from build123d import *
from build123d.topology import SkipClean

# Parameters (mm, degrees)
SKETCH_1_R               = 8
EXTRUDE_1_DEPTH          = 17
SKETCH_2_R               = 30
EXTRUDE_2_DEPTH          = 3
CUT_EXTRUDE_1_DEPTH      = 47.904158
CUT_EXTRUDE_2_DEPTH      = 50.558047
CUT_EXTRUDE_2_DEPTH_BACK = 50.558047
SKETCH_4_R               = 1.15
EXTRUDE_START            = 15
EXTRUDE_3_DEPTH          = 15
FILLET_1_R               = 3
CUT_EXTRUDE_3_DEPTH      = 46.70558
CUT_EXTRUDE_3_DEPTH_BACK = 46.70558
SKETCH_6_R               = 1.25


with BuildPart() as part:
    # 草图1 → 凸台-拉伸1 (new body)
    with BuildSketch(Plane(origin=(0, 0, 0), x_dir=(1, 0, 0), z_dir=(0, 1, 0))):
        with Locations(Location((0, 0, 0), (0, 0, 270))):
            Circle(SKETCH_1_R)
    extrude(amount=EXTRUDE_1_DEPTH)

    # 草图2 → 凸台-拉伸2 (add)
    with BuildSketch(Plane(origin=(0, 17, 0), x_dir=(1, 0, 0), z_dir=(0, 1, 0))):
        with Locations(Location((0, 0, 0), (0, 0, 270))):
            Circle(SKETCH_2_R)
    extrude(amount=EXTRUDE_2_DEPTH)

    # 草图3 → 切除-拉伸1 (cut, through all)
    with BuildSketch(Plane.XZ):
        with BuildLine():
            Line((-4, 3), (-4, -3))
            ThreePointArc((-4, -3), (5, 0), (-4, 3))
        make_face()
    extrude(amount=-CUT_EXTRUDE_1_DEPTH, mode=Mode.SUBTRACT)

    # 草图4 → 切除-拉伸2 (cut, two sides: drawn at the far end of the back side and taken through both)
    with BuildSketch(Plane(origin=(-4, 0, 0), x_dir=(0, 0, -1), z_dir=(1, 0, 0)).offset(-CUT_EXTRUDE_2_DEPTH_BACK)):
        with Locations((0, 10)):
            Circle(SKETCH_4_R)
    extrude(amount=CUT_EXTRUDE_2_DEPTH + CUT_EXTRUDE_2_DEPTH_BACK, mode=Mode.SUBTRACT)

    # 草图5 → 凸台-拉伸3 (add)
    with SkipClean():  # the faces are left unmerged after this step: merging them gives an invalid solid
        with BuildSketch(Plane.XZ.offset(-17).offset(EXTRUDE_START)):
            with BuildLine():
                Line((-2, 29.933259), (-2, 20))
                Line((-2, 20), (2, 20))
                Line((2, 20), (2, 29.933259))
                ThreePointArc((2, 29.933259), (0, 30), (-2, 29.933259))
            make_face()
        extrude(amount=-EXTRUDE_3_DEPTH)

    # 圆角1
    fillet_1_edges = [part.edges().sort_by_distance(p)[0] for p in [
        (0, 17, -8),
    ]]
    fillet(fillet_1_edges, radius=FILLET_1_R)

    # 草图6 → 切除-拉伸3 (cut, two sides: drawn at the far end of the back side and taken through both)
    with SkipClean():  # the faces are left unmerged after this step: merging them gives an invalid solid
        with BuildSketch(Plane.XZ.offset(-17).offset(-CUT_EXTRUDE_3_DEPTH_BACK)):
            with Locations(Location((-16, 0, 0), (0, 0, 270))):
                Circle(SKETCH_6_R)
            with Locations(Location((16, 0, 0), (0, 0, 90))):
                Circle(SKETCH_6_R)
        extrude(amount=CUT_EXTRUDE_3_DEPTH + CUT_EXTRUDE_3_DEPTH_BACK, mode=Mode.SUBTRACT)


solid = part.part
Verification items for the finished model (mm, model axes). A direction names the side the tool comes from. Coordinates: 2 decimals unless noted, no trailing zeros. Write each loop counter-clockwise with the first axis right and the second up, starting at its lowest first coordinate (ties: lowest second). Pieces come first, ordered by that corner, then holes. Notation, with made-up numbers: M 70,-20.5 L 114,-20.5 A10 cw 114,-14.5 Z; hole C -39.5,46 d4. An arc over 180 degrees is marked long. Use CSV: the item, a comma, the result in double quotes.
Q1. Go/stop test with flat-tipped pins: P1, Ø1, axis at x = 7.5, y = 9, coming from the -Z side; P2, Ø4, axis at x = -16, z = 0, coming from the -Y side; P3, Ø10, axis at y = 17, z = 10, coming from the +X side. Record where each tip stops, or that it passes through.
Computed values:
P1,"z = -3.87"
P2,"y = 17"
P3,"x = 29.58"
Q2. Section check A-A, the plane z = 0. State how many separate pieces and enclosed holes the cut face has, and give its area (3 significant figures).
Computed values:
separate pieces,"6"
enclosed holes,"0"
area,"245 mm²"
Q3. Set-up check for faces 4 (the flat face through (2, 9, 25)), 5 (the cylindrical face through (-7.81, 6.9, -1.73)), 6 (the flat face through (-2, 9, 25)), 7 (the flat face through (0, 2, 25)), 8 (the flat face through (-4, 9.9, -1.3)): record each of +Z, -Z, +X, -X, +Y, -Y from which the full face is reachable in a straight line by a thin tool's end or side.
Computed values:
face 4,"+Z, +X, -Y"
face 5,"-Y"
face 6,"+Z, -X, -Y"
face 7,"+Z, +X, -X, -Y"
face 8,"+Y, -Y"
Q4. Section check B-B, the plane x = 0. Enter the section's corners in (y, z).
Computed values:
outline,"M 0,-8 L 14,-8 A3 cw 17,-11 L 17,-30 L 20,-30 L 20,-5 L 0,-5 Z; M 0,5 L 20,5 L 20,30 L 2,30 L 2,20 L 17,20 L 17,11 A3 cw 14,8 L 0,8 Z"
Q5. Section check D-D, the plane y = 10. Enter the section's corners in (x, z), and give its area (3 significant figures).
Computed values:
outline,"M -7.92,-1.15 A8 ccw 7.92,-1.15 L 4.87,-1.15 A5 cw -4,-3 L -4,-1.15 Z; M -7.92,1.15 L -4,1.15 L -4,3 A5 cw 4.87,1.15 L 7.92,1.15 A8 ccw Z; M -2,20 L 2,20 L 2,29.93 A30 ccw -2,29.93 Z"
area,"150 mm²"
Q6. Mould release check, pull along Y, two halves, no side actions. Record for faces 1 (the cylindrical face through (6.41, 8.877, 0.249)), 2 (the flat face through (-5, 0, 0)), 3 (the flat face through (0, 9, 20)): pulls with the +Y half, pulls with the -Y half, needs draft (parallel to the pull), parting line crosses it, or undercut.
Computed values:
face 1,"undercut"
face 2,"pulls with the -Y half"
face 3,"needs draft"
Q7. Thickness scan on line 1 along X through (y, z) = (18.3, 0); line 2 along X through (y, z) = (17.75, -1); line 3 along Y through (x, z) = (9.5, 22). Record the ranges inside material, lowest first. Write a range as [from, to].
Computed values:
line 1,"[-30, -17.25], [-14.75, -4], [5, 14.75], [17.25, 30]"
line 2,"[-29.98, -16.75], [-15.25, -4], [4.9, 15.25], [16.75, 29.98]"
line 3,"[17, 20]"
Q8. Section check C-C, the plane y = 14.75. Enter the section's corners in (x, z).
Computed values:
outline,"C 0,0 d16.19; M -2,20 L 2,20 L 2,29.93 A30 ccw -2,29.93 Z; hole M -4,-3 A5 ccw long -4,3 Z"
